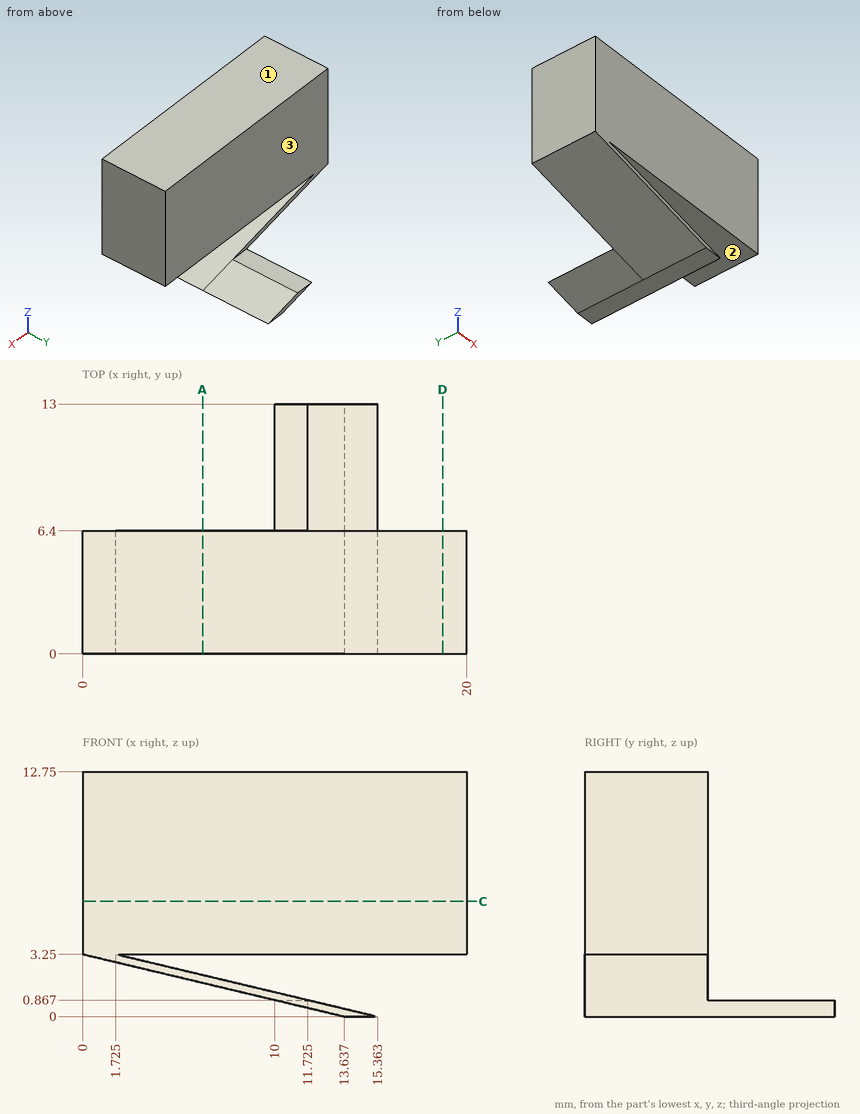
The drawing under review shows one solid part. Ordinate dimensions are in mm from its lowest x, y, z. Give positions to 0.01 mm unless a question says otherwise; leave off trailing zeros. Write each loop counter-clockwise with the first axis right and the second up, starting at its lowest first coordinate (ties: lowest second). Pieces come first, ordered by that corner, then holes.
1. Wall thickness on L1, parallel to Y at x = 2, z = 9; L2, parallel to Z at x = 10.25, y = 6; L3, parallel to Z at x = 5, y = 1.5: over which ranges is each line inside the solid? List them lowest first.
2. Add section A-A, the plane x = 6.25. Write out the cut boundary in (y, z).
3. For P1, Ø3.5, axis at x = 10, z = 7, coming from the +Y side; P2, Ø6, axis at x = 8, y = 7.5, coming from the -Z side; P3, Ø5, axis at x = 7.5, y = 4, coming from the -Z side, all flat-tipped, find the tip position at first contact; note any pin that passes through.
4. Add section D-D, the plane x = 18.75. Write out the cut boundary in (y, z).
5. Add section C-C, the plane z = 6. Write out the cut boundary in (x, y), plus the area to 3 significant figures.
6. Draft analysis for pull direction Z (two halves, no side actions). For the marked faces 1, 2 and 3, state which applies: +Z half, -Z half, draft (parallel to the pull), parting line (faces both ways), or undercut.
Worked answers:
1. L1: y = 0 to 6.4
1. L2: z = 0.81 to 1.22, 3.25 to 12.75
1. L3: z = 2.06 to 2.47, 3.25 to 12.75
2. outline: (0, 1.76) - (6.4, 1.76) - (6.4, 2.17) - (0, 2.17) - close; (0, 3.25) - (6.4, 3.25) - (6.4, 12.75) - (0, 12.75) - close
3. P1: stops at y = 6.4
3. P2: stops at z = 0.63
3. P3: stops at z = 0.87
4. outline: (0, 3.25) - (6.4, 3.25) - (6.4, 12.75) - (0, 12.75) - close
5. outline: (0, 0) - (20, 0) - (20, 6.4) - (0, 6.4) - close
5. area: 128 mm2
6. face 1: +Z half
6. face 2: undercut
6. face 3: draft
